The listing builds one solid part. Answer for the finished solid, in the listing's coordinates (mm). A direction names the side the tool comes from. Give positions to 0.01 mm unless a question says otherwise; leave off trailing zeros. Order: outer loops, then holes, each group sorted by start corner. A loop starts at its lowest first (then second) coordinate and runs counter-clockwise, first axis right, second up. Notation, with made-up numbers: (-20.5, 45.25) - (34.5, 45.25) arc R31 ccw to (34.5, 79.25) - close; hole circle Ø3 at (52, 28). An arc over 180 degrees is marked (long way). Answer in a Markdown table with one row per item.
from build123d import *

# Parameters (mm, degrees)
F1_DEPTH       = 7.9375
F3_DEPTH       = 22.225
F4_R           = 6.35
F5_DEPTH       = 2.38125
F8_R           = 7.239
F9_DEPTH       = 4.7625
F10_R          = 6.477
F11_DEPTH      = 3.175
F12_R          = 7.3025
F13_DEPTH      = 3.175
F14_R          = 0.79375
F15_DEPTH      = 8.7998181024
F15_DEPTH_BACK = 8.7998181024


with BuildPart() as f1:
    # F0 (on Top) → F1 (new body)
    with BuildSketch(Plane.XY):
        Polygon((8.7988181024, 5.08), (0, 10.16), (-8.7988181024, 5.08), (-8.7988181024, -5.08), (0, -10.16), (8.7988181024, -5.08), align=None)
    extrude(amount=F1_DEPTH)

    # F2 (on face) → F3 (join)
    with BuildSketch(Plane.XY.offset(7.9375)):
        Polygon((1.905, 7.2003333051), (0, 8.7988181024), (-1.905, 7.2003333051), align=None)
        Polygon((-5.2831715579, 5.2499450467), (-7.62, 4.3994090512), (-7.1881715579, 1.9503882583), align=None)
        Polygon((-7.1881715579, -1.9503882583), (-7.62, -4.3994090512), (-5.2831715579, -5.2499450467), align=None)
        Polygon((-1.905, -7.2003333051), (0, -8.7988181024), (1.905, -7.2003333051), align=None)
        Polygon((5.2831715579, -5.2499450467), (7.62, -4.3994090512), (7.1881715579, -1.9503882583), align=None)
        Polygon((7.1881715579, 1.9503882583), (7.62, 4.3994090512), (5.2831715579, 5.2499450467), align=None)
    extrude(amount=F3_DEPTH)

    # F4 (on face) → F5 (join)
    with BuildSketch(Plane.XY.offset(30.1625)):
        Polygon((8.7988181024, 5.08), (0, 10.16), (-8.7988181024, 5.08), (-8.7988181024, -5.08), (0, -10.16), (8.7988181024, -5.08), align=None)
        Circle(F4_R, mode=Mode.SUBTRACT)
    extrude(amount=F5_DEPTH)

    # F6 (on Right) → F7 (revolve)
    with BuildSketch(Plane.YZ):
        with BuildLine():
            Line((-6.477, 34.925), (0, 34.925))
            Line((0, 34.925), (0, 40.48125))
            ThreePointArc((0, 40.48125), (-5.6126600757, 38.1564100757), (-7.9375, 32.54375))
            Line((-7.9375, 32.54375), (-6.477, 32.54375))
            Line((-6.477, 32.54375), (-6.477, 34.925))
        make_face()
    revolve(axis=Axis((0, 0, 32.54375), (0, 0, 1)))

    # F8 (on face) → F9 (cut)
    with BuildSketch(Plane(origin=(0, 0, 0), x_dir=(1, 0, 0), z_dir=(0, 0, -1))):
        Circle(F8_R)
    extrude(amount=-F9_DEPTH, mode=Mode.SUBTRACT)

    # F10 (on face) → F11 (cut, through all)
    with BuildSketch(Plane(origin=(0, 0, 4.7625), x_dir=(1, 0, 0), z_dir=(0, 0, -1))):
        Circle(F10_R)
    extrude(amount=-F11_DEPTH, mode=Mode.SUBTRACT)

    # F12 (on face) → F13 (join)
    with BuildSketch(Plane(origin=(0, 0, 0), x_dir=(1, 0, 0), z_dir=(0, 0, -1))):
        Polygon((-8.1114104382, -4.683125), (0, -9.36625), (8.1114104382, -4.683125), (8.1114104382, 4.683125), (0, 9.36625), (-8.1114104382, 4.683125), align=None)
        Circle(F12_R, mode=Mode.SUBTRACT)
    extrude(amount=F13_DEPTH)

    # F14 (on Right) → F15 (cut, two sides)
    with BuildSketch(Plane.YZ) as f15_sk:
        with Locations((0, 38.95725)):
            Circle(F14_R)
    extrude(amount=-F15_DEPTH, mode=Mode.SUBTRACT)
    extrude(f15_sk.sketch, amount=F15_DEPTH_BACK, mode=Mode.SUBTRACT)


solid = f1.part
Item 1: Find section B-B on z = 31. Write down the section's boundary in (x, y), then the cut area to 3 significant figures.
Answer block:
| item | result |
|---|---|
| outline | (-8.8, -5.08) - (0, -10.16) - (8.8, -5.08) - (8.8, 5.08) - (0, 10.16) - (-8.8, 5.08) - close; hole circle Ø12.7 at (0, 0) |
| area | 142 mm² |
Item 2: Find section C-C on x = 2.75. Count the separate pieces of the cut face and the enclosed holes in it, then the cut area to 3 significant figures.
Answer block:
| item | result |
|---|---|
| separate pieces | 3 |
| enclosed holes | 1 |
| area | 112 mm² |
Item 3: Consider line 1 (Z direction, x = -4.25, y = 7); line 2 (X direction, y = 0, z = 2.2); line 3 (Y direction, x = 0, z = -1.15). Determine where each line is inside the solid, lowest interval first.
Answer block:
| item | result |
|---|---|
| line 1 | 0 to 7.94, 30.16 to 32.54 |
| line 2 | -8.8 to -7.24, 7.24 to 8.8 |
| line 3 | -9.37 to -7.3, 7.3 to 9.37 |
Item 4: Which of the six approach directions +Z, -Z, +X, -X, +Y, -Y give full straight-line access (tool end or side, diameter ignored) to faces 4 (the face through (6.47, 4.82, 18.89)), 5 (the face through (7.4, 3.16, 18.89)), 6 (the face through (-7.2, -3.7, 32.544)), 7 (the face through (6.44, -4.83, 18.89)), 8 (the face through (-0.942, -7.177, 2.348))?
Answer block:
| item | result |
|---|---|
| face 4 | +X, +Y |
| face 5 | +X |
| face 6 | +Z |
| face 7 | +X, -Y |
| face 8 | -Z |
Item 5: Find section A-A on z = 10. Write down the section's boundary in (x, y) (3 decimals), then the cut area to 3 significant figures.
Answer block:
| item | result |
|---|---|
| outline | (-7.62, -4.399) - (-5.283, -5.25) - (-7.188, -1.95) - close; (-7.62, 4.399) - (-7.188, 1.95) - (-5.283, 5.25) - close; (-1.905, -7.2) - (0, -8.799) - (1.905, -7.2) - close; (-1.905, 7.2) - (1.905, 7.2) - (0, 8.799) - close; (5.283, -5.25) - (7.62, -4.399) - (7.188, -1.95) - close; (5.283, 5.25) - (7.188, 1.95) - (7.62, 4.399) - close |
| area | 18.3 mm² |
Item 6: Determine the mould class of faces 1 (the face through (-4.338, 7.656, 3.913)), 2 (the face through (-6.323, 1.404, 33.751)), 3 (the face through (-8.799, 0, 31)) for opening direction Y: pulls with the +Y half, pulls with the -Y half, needs draft (parallel to the pull), parting line crosses it, or undercut.
Answer block:
| item | result |
|---|---|
| face 1 | pulls with the +Y half |
| face 2 | undercut |
| face 3 | needs draft |
Item 7: Each of these flat-tipped pins is pushed along its axis until it touches: P1, Ø5, axis at y = 4.5, z = 12.5, coming from the -X side; P2, Ø8, axis at x = 6.5, z = 8.5, coming from the +Y side; P3, Ø1.5, axis at x = 6, z = 12.5, coming from the +Y side; P4, Ø1, axis at x = 3, z = 8.5, coming from the -Y side. Where does it stop, or does it pass through?
Answer block:
| item | result |
|---|---|
| P1 | x = -7.62 |
| P2 | y = 8.69 |
| P3 | y = 5.25 |
| P4 | through |
